Work out the finished part from the listing and answer in its coordinate system (mm). Give positions to 0.01 mm unless a question says otherwise; leave off trailing zeros. Write each loop counter-clockwise with the first axis right and the second up, starting at its lowest first coordinate (ties: lowest second). Pieces come first, ordered by that corner, then holes. Notation, with made-up numbers: (57.5, 77) - (104.5, 77) arc R32 ccw to (104.5, 115) - close; hole circle Ø3 at (18, 77). An arc over 180 degrees is marked (long way). Write item = value, one per line.
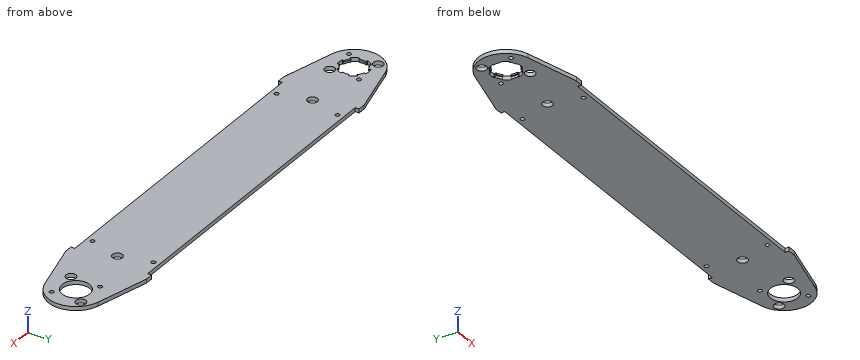
from build123d import *

# Parameters (mm, degrees)
F0_R     = 1.7272
F0_R_2   = 3.96875
F0_R_3   = 10.31875
F0_R_4   = 11.1125
F1_DEPTH = 3.175
F3_DEPTH = 3.175
F4_COUNT = 6
F4_ANGLE = 300
F5_R     = 11.1125
F6_DEPTH = 1.94945


with BuildPart() as f1:
    # F0 (on Top) → F1 (new body)
    with BuildSketch(Plane.XY):
        with BuildLine():
            Line((-303.6125627, 32.54375), (-346.1094200534, 21.5120031198))
            ThreePointArc((-346.1094200534, 21.5120031198), (-362.7501254, 0), (-346.1094200534, -21.5120031198))
            Line((-346.1094200534, -21.5120031198), (-303.6125627, -32.54375))
            Line((-303.6125627, -32.54375), (-297.2625627, -32.54375))
            Line((-297.2625627, -32.54375), (-297.2625627, -29.36875))
            Line((-297.2625627, -29.36875), (-43.2625627, -29.36875))
            Line((-43.2625627, -29.36875), (-43.2625627, -32.54375))
            Line((-43.2625627, -32.54375), (-36.9125627, -32.54375))
            Line((-36.9125627, -32.54375), (5.5842946534, -21.5120031198))
            ThreePointArc((5.5842946534, -21.5120031198), (22.225, 0), (5.5842946534, 21.5120031198))
            Line((5.5842946534, 21.5120031198), (-36.9125627, 32.54375))
            Line((-36.9125627, 32.54375), (-43.2625627, 32.54375))
            Line((-43.2625627, 32.54375), (-43.2625627, 29.36875))
            Line((-43.2625627, 29.36875), (-297.2625627, 29.36875))
            Line((-297.2625627, 29.36875), (-297.2625627, 32.54375))
            Line((-297.2625627, 32.54375), (-303.6125627, 32.54375))
        make_face()
        with Locations((-282.9750627, -24.60625)):
            Circle(F0_R, mode=Mode.SUBTRACT)
        with Locations((-352.3117115589, -11.7865861589)):
            Circle(F0_R, mode=Mode.SUBTRACT)
        with Locations((-328.7385392411, -11.7865861589)):
            Circle(F0_R_2, mode=Mode.SUBTRACT)
        with Locations((-57.5500627, -24.60625)):
            Circle(F0_R, mode=Mode.SUBTRACT)
        with Locations((-11.7865861589, -11.7865861589)):
            Circle(F0_R_2, mode=Mode.SUBTRACT)
        with Locations((11.7865861589, -11.7865861589)):
            Circle(F0_R, mode=Mode.SUBTRACT)
        with Locations((-340.5251254, 0)):
            Circle(F0_R_3, mode=Mode.SUBTRACT)
        with Locations((-289.7251254, 0)):
            Circle(F0_R_2, mode=Mode.SUBTRACT)
        with Locations((-352.3117115589, 11.7865861589)):
            Circle(F0_R_2, mode=Mode.SUBTRACT)
        with Locations((-328.7385392411, 11.7865861589)):
            Circle(F0_R, mode=Mode.SUBTRACT)
        with Locations((-282.9750627, 24.60625)):
            Circle(F0_R, mode=Mode.SUBTRACT)
        with Locations((-50.8, 0)):
            Circle(F0_R_2, mode=Mode.SUBTRACT)
        Circle(F0_R_4, mode=Mode.SUBTRACT)
        with Locations((-11.7865861589, 11.7865861589)):
            Circle(F0_R, mode=Mode.SUBTRACT)
        with Locations((11.7865861589, 11.7865861589)):
            Circle(F0_R_2, mode=Mode.SUBTRACT)
        with Locations((-57.5500627, 24.60625)):
            Circle(F0_R, mode=Mode.SUBTRACT)
    extrude(amount=F1_DEPTH)

    # F2 (on face) → F3 (cut, through all)
    with BuildSketch(Plane(origin=(0, 0, 0), x_dir=(1, 0, 0), z_dir=(0, 0, -1))):
        with BuildLine():
            ThreePointArc((-347.8215834984, -7.2964580984), (-349.4614250353, -5.159375), (-350.49227252, -2.6706890217))
            Line((-350.49227252, -2.6706890217), (-352.0256797693, -3.0815642558))
            ThreePointArc((-352.0256797693, -3.0815642558), (-350.8362403638, -5.953125), (-348.9441155135, -8.4189901135))
            Line((-348.9441155135, -8.4189901135), (-347.8215834984, -7.2964580984))
        make_face()
    f3 = extrude(amount=-F3_DEPTH, mode=Mode.SUBTRACT)

    # F4: F3 ×6 about axis
    f4_axis = Axis((-340.5251254, 0, 0), (0, 0, -1))
    for i in range(1, F4_COUNT):
        add(f3.rotate(f4_axis, i * F4_ANGLE / (F4_COUNT - 1)), mode=Mode.SUBTRACT)

    # F5 (on face) → F6 (cut)
    with BuildSketch(Plane(origin=(0, 0, 0), x_dir=(1, 0, 0), z_dir=(0, 0, -1))):
        with Locations((-340.5251254, 0)):
            Circle(F5_R)
    extrude(amount=-F6_DEPTH, mode=Mode.SUBTRACT)


solid = f1.part
1. Given pin 1 (1 mm diameter, centred on x = -286, z = 0.5, fed in from -Y); pin 2 (0.6 mm diameter, centred on x = -330.5, y = 1.5, fed in from -Z); pin 3 (3 mm diameter, centred on x = -282.98, y = -24.61, fed in from +Z); pin 4 (1.6 mm diameter, centred on x = -140, z = 1.5, fed in from +Y), each flat-ended and moving along its own axis, determine where each tip first touches the part or whether it passes through.
Solution:
pin_1 = -29.37
pin_2 = 1.95
pin_3 = through
pin_4 = 29.37
2. Find section B-B, the plane x = -235. Give the vertices of the cut face in (y, z) (3 decimals).
Solution:
outline = (-29.369, 0) - (29.369, 0) - (29.369, 3.175) - (-29.369, 3.175) - close
3. Find section C-C, the plane x = 0. Give the vertices of the cut face in (y, z) (1 decimal), then the cut area to 3 significant figures.
Solution:
outline = (-23, 0) - (-11.1, 0) - (-11.1, 3.2) - (-23, 3.2) - close; (11.1, 0) - (23, 0) - (23, 3.2) - (11.1, 3.2) - close
area = 75.2 mm^2
4. Find section A-A, the plane x = -50.8. Give the vertices of the cut face in (y, z) (3 decimals).
Solution:
outline = (-29.369, 0) - (-3.969, 0) - (-3.969, 3.175) - (-29.369, 3.175) - close; (3.969, 0) - (29.369, 0) - (29.369, 3.175) - (3.969, 3.175) - close
5. Straight lines are drawn through the part: line 1 (X direction, y = 1, z = 2.6); line 2 (X direction, y = -12.5, z = 1.4); line 3 (Y direction, x = -265.5, z = 1.3). For each, find the intervals that lie inside material, in ascending order.
Solution:
line_1 = -362.73 to -350.8, -330.25 to -293.57, -285.88 to -54.64, -46.96 to -11.07, 11.07 to 22.2
line_2 = -358.9 to -353.88, -350.74 to -332.64, -324.83 to -15.69, -7.88 to 10.21, 13.36 to 18.38
line_3 = -29.37 to 29.37
6. Find section D-D, the plane x = -309. Give the vertices of the cut face in (y, z) (3 decimals), then the cut area to 3 significant figures.
Solution:
outline = (-31.145, 0) - (31.145, 0) - (31.145, 3.175) - (-31.145, 3.175) - close
area = 198 mm^2
